```python
from build123d import *

# Parameters (mm, degrees)
SKETCH_1_R      = 40.9
SKETCH_1_R_2    = 1.525
EXTRUDE_1_DEPTH = 1.5
EXTRUDE_3_DEPTH = 1.5
FILLET_1_R      = 2
SKETCH_3_W      = 30
SKETCH_3_H      = 5
EXTRUDE_4_DEPTH = 1.5


with BuildPart() as part:
    # 草图1 → 凸台-拉伸1 (new body)
    with BuildSketch(Plane(origin=(0, 0, 0), x_dir=(1, 0, 0), z_dir=(0, 1, 0))):
        with BuildLine():
            Line((-46.9, 0), (-46.9, 46.9))
            Line((-46.9, 46.9), (-16.9, 46.9))
            Line((-16.9, 46.9), (-16.9, 46.574671228))
            ThreePointArc((-16.9, 46.574671228), (-16.079234093, 44.95930534), (-14.290593047, 44.669776699))
            ThreePointArc((-14.290593047, 44.669776699), (37.88033008, -27.65303949), (-46.9, 0))
        make_face()
        Circle(SKETCH_1_R, mode=Mode.SUBTRACT)
        with Locations((-19.9, 39.130550724)):
            Circle(SKETCH_1_R_2, mode=Mode.SUBTRACT)
        with Locations((0, 43.9)):
            Circle(SKETCH_1_R_2, mode=Mode.SUBTRACT)
        with Locations((43.9, 0)):
            Circle(SKETCH_1_R_2, mode=Mode.SUBTRACT)
        with Locations((0, -43.9)):
            Circle(SKETCH_1_R_2, mode=Mode.SUBTRACT)
        with Locations((-43.9, 0)):
            Circle(SKETCH_1_R_2, mode=Mode.SUBTRACT)
        with Locations((-43.9, 39.130550724)):
            Circle(SKETCH_1_R_2, mode=Mode.SUBTRACT)
    extrude(amount=EXTRUDE_1_DEPTH)

    # 草图2 → 凸台-拉伸3 (add)
    with BuildSketch(Plane(origin=(0, 0, 0), x_dir=(1, 0, 0), z_dir=(0, 1, 0))):
        with BuildLine():
            Line((-37.06798849, 17.285086905), (-33.052288278, 15.412535144))
            ThreePointArc((-33.052288278, 15.412535144), (-31.934408281, 15.352211673), (-31.08609948, 16.082736681))
            ThreePointArc((-31.08609948, 16.082736681), (-23.380571231, 26.04513177), (-12.647507481, 32.634959086))
            ThreePointArc((-12.647507481, 32.634959086), (-12.090765455, 33.012479837), (-11.754991898, 33.595351795))
            Line((-11.754991898, 33.595351795), (-9.89460553, 39.685095205))
            ThreePointArc((-9.89460553, 39.685095205), (-26.015599209, 31.559445461), (-37.06798849, 17.285086905))
        make_face()
    extrude(amount=EXTRUDE_3_DEPTH)

    # 圆角1
    fillet_1_edges = [part.edges().sort_by_distance(p)[0] for p in [
        (-9.89460553, 0.75, -39.685095205),
        (-37.06798849, 0.75, -17.285086905),
    ]]
    fillet(fillet_1_edges, radius=FILLET_1_R)

    # 草图3 → 凸台-拉伸4 (add)
    with BuildSketch(Plane(origin=(0, 1.5, 0), x_dir=(1, 0, 0), z_dir=(0, 1, 0))):
        with Locations((-31.9, 49.4)):
            Rectangle(SKETCH_3_W, SKETCH_3_H)
    extrude(amount=-EXTRUDE_4_DEPTH)


solid = part.part
```
Could you check a few things on this model? Use its own coordinates, in mm. A direction names the side the tool comes from. Coordinates: 2 decimals unless noted, no trailing zeros. Write each loop counter-clockwise with the first axis right and the second up, starting at its lowest first coordinate (ties: lowest second). Pieces come first, ordered by that corner, then holes. Notation, with made-up numbers: M -25,42 L -2,42 A4 cw -2,49 Z; hole C -13,5.25 d1. An arc over 180 degrees is marked long. Answer as CSV lines item,"result". Start each with the question number.
1) We'd pull the mould along X, two halves only. Please class faces 1 (the cylindrical face through (-42.445, 0.74, -0.458)), 2 (the flat face through (-21.1, 0, -28.3)): +X half, -X half, draft (parallel to the pull), parting line (faces both ways), or undercut.
2) I want a section at A-A, the plane z = 13. Please give me the cut outline in (x, y), and give its area (3 significant figures).
3) Please list where these lines run through material, in increasing order: line 1 (Z direction, x = 0, y = 0.6) (3 decimals); line 2 (Z direction, x = -19.9, y = 0.9). Write a range as from..to.
4) For faces 3 (the cylindrical face through (-23.51, 0.74, -25.93)), 4 (the flat face through (-21.1, 1.5, -28.3)), which set-ups out of +Z, -Z, +X, -X, +Y, -Y let a thin tool reach every point of the face, with its end or its side?
5) I want a section at B-B, the plane x = 21.5. Please give me the cut outline in (y, z), and give its area (3 significant figures).
6) I want a section at C-C, the plane y = 1.15. Give the number of separate pieces and of enclosed holes in the cut face, and give its area (3 significant figures).
7) I want a section at D-D, the plane x = -19.9. Please give me the cut outline in (y, z).
Data:
1,face 1,"undercut"
1,face 2,"draft"
2,outline,"M -45.06,0 L -38.78,0 L -38.78,1.5 L -45.06,1.5 Z; M 38.78,0 L 45.06,0 L 45.06,1.5 L 38.78,1.5 Z"
2,area,"18.8 mm^2"
3,line 1,"z = -46.9..-45.425, -42.375..-40.9, 40.9..42.375, 45.425..46.9"
3,line 2,"z = -51.9..-40.66, -37.61..-28.79, 35.73..42.47"
4,face 3,"+Y, -Y"
4,face 4,"+Z, -Z, +X, -X, +Y"
5,outline,"M 0,-41.68 L 1.5,-41.68 L 1.5,-34.79 L 0,-34.79 Z; M 0,34.79 L 1.5,34.79 L 1.5,41.68 L 0,41.68 Z"
5,area,"20.7 mm^2"
6,separate pieces,"1"
6,enclosed holes,"7"
6,area,"2,410 mm^2"
7,outline,"M 0,-51.9 L 1.5,-51.9 L 1.5,-40.66 L 0,-40.66 Z; M 0,-37.61 L 1.5,-37.61 L 1.5,-28.79 L 0,-28.79 Z; M 0,35.73 L 1.5,35.73 L 1.5,42.47 L 0,42.47 Z"
